Answer from the drawing. Dimensions are ordinates in mm from the lowest x, y and z of the part. A direction names the side the tool comes from. Give positions to 0.01 mm unless a question says otherwise; leave off trailing zeros. Loops run counter-clockwise (first coordinate to the right, second up) from the corner with the lowest first, then second, coordinate; pieces in that order, holes last. Notation, with made-up numbers: M 62,-21 L 102,-21 A34 ccw 102,11 Z; hole C 39.25,84.5 d5. An arc over 180 degrees is marked long. Use a Markdown table: item, result.
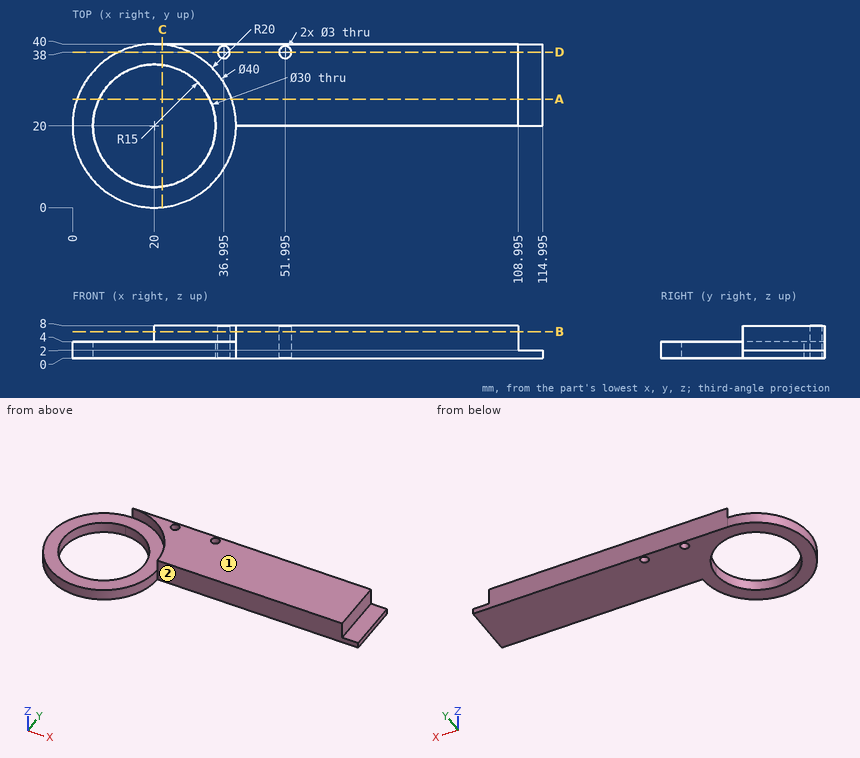
(1) A cutting plane is placed at A-A (y = 26.5). Write down the section's boundary in (x, z) (1 decimal), and give its area (3 significant figures).
Entries:
| item | result |
|---|---|
| outline | M 1.1,0 L 6.5,0 L 6.5,4 L 1.1,4 Z; M 33.5,0 L 115,0 L 115,2 L 109,2 L 109,8 L 38.9,8 L 38.9,4 L 33.5,4 Z |
| area | 616 mm² |
(2) A cutting plane is placed at B-B (z = 6.5). Write down the section's boundary in (x, y) (1 decimal), and give its area (3 significant figures).
Entries:
| item | result |
|---|---|
| outline | M 20,40 A20 cw 40,20 L 109,20 L 109,40 Z; hole C 37,38 d3; hole C 52,38 d3 |
| area | 1,450 mm² |
(3) A cutting plane is placed at C-C (x = 22). Write down the section's boundary in (y, z).
Entries:
| item | result |
|---|---|
| outline | M 0.1,0 L 5.13,0 L 5.13,4 L 0.1,4 Z; M 34.87,0 L 40,0 L 40,8 L 39.9,8 L 39.9,4 L 34.87,4 Z |
(4) Which of the six approach directions +Z, -Z, +X, -X, +Y, -Y give full straight-line access (tool end or side, diameter ignored) to the marked faces 1 and 2?
Entries:
| item | result |
|---|---|
| face 1 | +Z, +X, -X, +Y, -Y |
| face 2 | +Z, -Z, +X, -Y |
(5) Given P1, Ø1.8, axis at y = 27, z = 5.5, coming from the +X side (1 decimal); P2, Ø5, axis at x = 49.5, y = 34, coming from the -Z side; P3, Ø1.8, axis at x = 112, y = 27, coming from the +Z side; P4, Ø1, axis at x = 45, z = 1, coming from the -Y side, each flat-ended and moving along its own axis, determine where each tip first touches the part or whether it passes through.
Entries:
| item | result |
|---|---|
| P1 | stops at x = 109 |
| P2 | stops at z = 0 |
| P3 | stops at z = 2 |
| P4 | stops at y = 20 |
(6) Consider probe 1 along Y at (x, z) = (42.5, 6); probe 2 along Z at (x, y) = (22.5, 5); probe 3 along X at (y, z) = (23.5, 1.25) (1 decimal). Determine where each line is inside the solid, lowest interval first. Write a range as [from, to].
Entries:
| item | result |
|---|---|
| probe 1 | y = [20, 40] |
| probe 2 | z = [0, 4] |
| probe 3 | x = [0.3, 5.4], [34.6, 115] |
(7) A cutting plane is placed at D-D (y = 38). Write down the section's boundary in (x, z) (1 decimal).
Entries:
| item | result |
|---|---|
| outline | M 11.3,0 L 35.5,0 L 35.5,8 L 28.7,8 L 28.7,4 L 11.3,4 Z; M 38.5,0 L 50.5,0 L 50.5,8 L 38.5,8 Z; M 53.5,0 L 115,0 L 115,2 L 109,2 L 109,8 L 53.5,8 Z |
